Build history of the part. All positions in model axes, mm. A direction names the side the tool comes from. Give positions to 0.01 mm unless a question says otherwise; leave off trailing zeros. Loops run counter-clockwise (first coordinate to the right, second up) from the corner with the lowest first, then second, coordinate; pieces in that order, holes last. Notation, with made-up numbers: M 38.5,16 L 49.5,16 A24 cw 49.5,50 Z; hole C 81.5,43 d1. An arc over 180 degrees is marked long. Answer as a JSON object with one key per item and string values. Group by question number.
1. Drill centre lines: line 1 along Y through (x, z) = (0, 4) (3 decimals); line 2 along Y through (x, z) = (0, -45) (3 decimals); line 3 along Y through (x, z) = (2, 365). Where is each one in solid material? Low to high. Write a range as [from, to].
2. Slice it at B-B (z = 36). List the corners of the cut face in (x, y) (3 decimals).
3. Slice it at D-D (x = -38.5). List the corners of the cut face in (y, z), then the cut area to 3 significant figures.
4. 3-axis set-ups, long thin cutter, end or side, ignore diameter. For faces 1 (the face through (-11.012, -49.592, 0.814)), 2 (the face through (-37.794, -28.979, 256.794)), 3 (the face through (-15.3, 45.4, 514.35)): which of +Z, -Z, +X, -X, +Y, -Y reach the whole face in a straight line?
5. Slice it at A-A (y = 0). List the corners of the cut face in (x, z) (3 decimals), then the cut area to 3 significant figures.
6. Slice it at C-C (x = 25). List the corners of the cut face in (y, z).
7. Drop flat-ended pins along their axis: pin 1 Ø12 at (x, y) = (-31, -29.5) entering from +Z; pin 2 Ø10 at (x, y) = (53, -5) entering from -Z; pin 3 Ø1 at (x, z) = (-14.5, 74.5) entering from -Y; pin 4 Ø3 at (x, y) = (52.24, 30.16) entering from +Z. Give the stop position or say it passes through.
8. Mould opens along Y. For faces 4 (the face through (-15.12, -11.59, -36)), 5 (the face through (-37.794, -28.979, 0.814)), 6 (the face through (-4, 16, -73.025)) say: released by +Y, released by -Y, zero draft, split by the parting line, or undercut.
from build123d import *

# Parameters (mm, degrees)
SKETCH1_R            = 19.05
SKETCH1_R_2          = 15.875
EXTRUDE1_DEPTH       = 6.35
EXTRUDE1_DEPTH_BACK  = 73.025
SKETCH1_4_R          = 47.625
SKETCH1_4_R_2        = 19.05
EXTRUDE3_DEPTH       = 6.35
SKETCH1_6_R          = 69.85
SKETCH1_6_R_2        = 50.8
SKETCH1_6_R_3        = 2.5796875
EXTRUDE5_DEPTH       = 6.35
SKETCH1_9_R          = 50.8
SKETCH1_9_R_2        = 47.625
EXTRUDE8_DEPTH       = 5.08
SKETCH1_10_R         = 50.8
SKETCH1_10_R_2       = 47.625
CUT_EXTRUDE1_DEPTH   = 1.651
SKETCH1_13_R         = 2.5796875
EXTRUDE9_DEPTH       = 6.35
SKETCH1_14_R         = 2.5796875
CUT_EXTRUDE5_DEPTH   = 6.35
CIRPATTERN1_COUNT    = 6
SKETCH5_R            = 50.8
SKETCH5_R_2          = 47.625
EXTRUDE11_DEPTH      = 508
EXTRUDE11_DEPTH_BACK = 1.651


with BuildPart() as part:
    # Sketch1 → Extrude1 (new body, two sides)
    with BuildSketch(Plane.XY) as extrude1_sk:
        Circle(SKETCH1_R)
        Circle(SKETCH1_R_2, mode=Mode.SUBTRACT)
    extrude(amount=EXTRUDE1_DEPTH)
    extrude(extrude1_sk.sketch, amount=-EXTRUDE1_DEPTH_BACK)

    # Sketch1_4 → Extrude3 (add)
    with BuildSketch(Plane.XY):
        Circle(SKETCH1_4_R)
        Circle(SKETCH1_4_R_2, mode=Mode.SUBTRACT)
    extrude(amount=EXTRUDE3_DEPTH)



with BuildPart() as body_2:
    # Sketch1_6 → Extrude5 (new body)
    with BuildSketch(Plane.XY):
        Circle(SKETCH1_6_R)
        Circle(SKETCH1_6_R_2, mode=Mode.SUBTRACT)
        with Locations((0, 60.325)):
            Circle(SKETCH1_6_R_3, mode=Mode.SUBTRACT)
    extrude(amount=EXTRUDE5_DEPTH)


with BuildPart() as part_1:
    add(part.part)

    add(body_2.part)  # Extrude8 merges body 2
    # Sketch1_9 → Extrude8 (add)
    with BuildSketch(Plane.XY):
        Circle(SKETCH1_9_R)
        Circle(SKETCH1_9_R_2, mode=Mode.SUBTRACT)
    extrude(amount=EXTRUDE8_DEPTH)

    # Sketch1_10 → Cut-Extrude1 (cut)
    with BuildSketch(Plane.XY):
        Circle(SKETCH1_10_R)
        Circle(SKETCH1_10_R_2, mode=Mode.SUBTRACT)
    extrude(amount=CUT_EXTRUDE1_DEPTH, mode=Mode.SUBTRACT)

    # Sketch1_13 → Extrude9 (add)
    with BuildSketch(Plane.XY):
        with Locations((0, 60.325)):
            Circle(SKETCH1_13_R)
    extrude(amount=EXTRUDE9_DEPTH)

    # Sketch1_14 → Cut-Extrude5 (cut)
    with BuildSketch(Plane.XY):
        with Locations((0, 60.325)):
            Circle(SKETCH1_14_R)
    cut_extrude5 = extrude(amount=CUT_EXTRUDE5_DEPTH, mode=Mode.SUBTRACT)

    # CirPattern1: Cut-Extrude5 ×6 about axis
    cirpattern1_axis = Axis((0, 0, 0), (0, 0, 1))
    for i in range(1, CIRPATTERN1_COUNT):
        add(cut_extrude5.rotate(cirpattern1_axis, i * 360 / CIRPATTERN1_COUNT), mode=Mode.SUBTRACT)

    # Sketch5 → Extrude11 (add, two sides)
    with BuildSketch(Plane.XY.offset(6.35)) as extrude11_sk:
        Circle(SKETCH5_R)
        Circle(SKETCH5_R_2, mode=Mode.SUBTRACT)
    extrude(amount=EXTRUDE11_DEPTH)
    extrude(extrude11_sk.sketch, amount=-EXTRUDE11_DEPTH_BACK)


solid = part_1.part
Established:
{
 "1": {"line 1": "y = [-69.85, -62.905], [-57.745, -15.875], [15.875, 57.745], [62.905, 69.85]", "line 2": "y = [-19.05, -15.875], [15.875, 19.05]", "line 3": "y = [-50.76, -47.58], [47.58, 50.76]"},
 "2": {"outline": "C 0,0 d101.6; hole C 0,0 d95.25"},
 "3": {"outline": "M -58.28,0 L -33.14,0 L -33.14,1.65 L -28.03,1.65 L -28.03,0 L 28.03,0 L 28.03,1.65 L 33.14,1.65 L 33.14,0 L 58.28,0 L 58.28,6.35 L 33.14,6.35 L 33.14,514.35 L 28.03,514.35 L 28.03,6.35 L -28.03,6.35 L -28.03,514.35 L -33.14,514.35 L -33.14,6.35 L -58.28,6.35 Z", "area": "5,910 mm^2"},
 "4": {"face 1": "-Z", "face 2": "+Z", "face 3": "+Z, +X, -X, +Y, -Y"},
 "5": {"outline": "M -69.85,0 L -50.8,0 L -50.8,1.651 L -47.625,1.651 L -47.625,0 L -19.05,0 L -19.05,-73.025 L -15.875,-73.025 L -15.875,6.35 L -47.625,6.35 L -47.625,514.35 L -50.8,514.35 L -50.8,6.35 L -69.85,6.35 Z; M 15.875,-73.025 L 19.05,-73.025 L 19.05,0 L 47.625,0 L 47.625,1.651 L 50.8,1.651 L 50.8,0 L 69.85,0 L 69.85,6.35 L 50.8,6.35 L 50.8,514.35 L 47.625,514.35 L 47.625,6.35 L 15.875,6.35 Z", "area": "4,360 mm^2"},
 "6": {"outline": "M -65.22,0 L -44.22,0 L -44.22,1.65 L -40.54,1.65 L -40.54,0 L 40.54,0 L 40.54,1.65 L 44.22,1.65 L 44.22,0 L 65.22,0 L 65.22,6.35 L 44.22,6.35 L 44.22,514.35 L 40.54,514.35 L 40.54,6.35 L -40.54,6.35 L -40.54,514.35 L -44.22,514.35 L -44.22,6.35 L -65.22,6.35 Z"},
 "7": {"pin 1": "stops at z = 514.35", "pin 2": "stops at z = 0", "pin 3": "stops at y = -48.83", "pin 4": "passes through"},
 "8": {"face 4": "split by the parting line", "face 5": "undercut", "face 6": "zero draft"}
}
